```python
from build123d import *

# Parameters (mm, degrees)
F0_W     = 84
F0_H     = 48.5
F0_W_2   = 0.8
F0_H_2   = 3.5
F1_DEPTH = 3
F2_START = 1.5
F2_DEPTH = 1.5


with BuildPart() as f1:
    # F0 (on Top) → F1 (new body)
    with BuildSketch(Plane.XY):
        with Locations((-0.0453250408, 1.1309052184)):
            Rectangle(F0_W, F0_H)
        with Locations((-41.2953250408, -20.5690947816)):
            Rectangle(F0_W_2, F0_H_2, mode=Mode.SUBTRACT)
        with Locations((41.2046749592, -20.5690947816)):
            Rectangle(F0_W_2, F0_H_2, mode=Mode.SUBTRACT)
        with Locations((-41.2953250408, 22.8309052184)):
            Rectangle(F0_W_2, F0_H_2, mode=Mode.SUBTRACT)
        with Locations((41.2046749592, 22.8309052184)):
            Rectangle(F0_W_2, F0_H_2, mode=Mode.SUBTRACT)
        with Locations((41.2046749592, -20.5690947816)):
            Rectangle(F0_W_2, F0_H_2)
        with Locations((41.2046749592, 22.8309052184)):
            Rectangle(F0_W_2, F0_H_2)
        with Locations((-41.2953250408, -20.5690947816)):
            Rectangle(F0_W_2, F0_H_2)
        with Locations((-41.2953250408, 22.8309052184)):
            Rectangle(F0_W_2, F0_H_2)
    extrude(amount=F1_DEPTH)

    # F0 (on Top) → F2 (cut)
    with BuildSketch(Plane.XY.offset(F2_START)):
        with Locations((-41.2953250408, -20.5690947816)):
            Rectangle(F0_W_2, F0_H_2)
        with Locations((-41.2953250408, 22.8309052184)):
            Rectangle(F0_W_2, F0_H_2)
        with Locations((41.2046749592, -20.5690947816)):
            Rectangle(F0_W_2, F0_H_2)
        with Locations((41.2046749592, 22.8309052184)):
            Rectangle(F0_W_2, F0_H_2)
    extrude(amount=F2_DEPTH, mode=Mode.SUBTRACT)


solid = f1.part
```
Geometry: final body of the model. Coordinates: model frame, mm. A direction names the side the tool comes from. Round coordinates to 2 decimals unless told otherwise and drop trailing zeros. Use one line per item in the form item = value.
Item 1: Draft query along Y for faces 3 (the flat face through (-1, 1, 0)), 4 (the flat face through (-1, -23.119, 1)), 5 (the flat face through (41.605, -21, 2)). Return one class per face: released by +Y, released by -Y, zero draft, split by the parting line, or undercut.
Evaluation:
face_3 = zero draft
face_4 = released by -Y
face_5 = undercut
Item 2: Contact query for a flat-ended pin moving along its axis: pin 1 Ø12 at (x, y) = (-0.5, 7.5) entering from -Z. Output: stop coordinate, or through.
Evaluation:
pin_1 = 0
Item 3: Access query for faces 1 (the flat face through (40.805, 23, 2)), 2 (the flat face through (-1, 25.381, 1)). Directions: +Z, -Z, +X, -X, +Y, -Y. A direction counts if a zero-diameter tool reaches every point of the face in a straight line with its end or side. Return the directions, or none.
Evaluation:
face_1 = +Z
face_2 = +Z, -Z, +X, -X, +Y
